The model under review builds one solid part; all positions refer to its coordinate system, in mm. A direction names the side the tool comes from. Round coordinates to 2 decimals unless told otherwise and drop trailing zeros. Order: outer loops, then holes, each group sorted by start corner. A loop starts at its lowest first (then second) coordinate and runs counter-clockwise, first axis right, second up. Notation, with made-up numbers: (-7, 78.5) -> (23, 78.5) arc R26 ccw to (23, 116.5) -> close; hole circle Ø4 at (-13, -16). An arc over 180 degrees is marked (long way). Use a Markdown table: item, result. Add a question column.
Autodesk Inventor part; units mm, degrees
ref_plane "YZ Plane" through (0, 0, 0) normal (1, 0, 0) x (0, 1, 0)
ref_plane "XZ Plane" through (0, 0, 0) normal (0, 1, 0) x (-1, 0, 0)
ref_plane "XY Plane" through (0, 0, 0) normal (0, 0, 1) x (1, 0, 0)
sketch "Sketch1" plane through (0, 0, 0) normal (0, 1, 0) x (-1, 0, 0)
  circle A0 centre (0, 0) radius 1
  circle A1 centre (0, 0) radius 2
  line L0 (2, 0) -> (-2, 0)
  line L1 (-2, 0) -> (-2, -8.25)
  line L2 (-2, -8.25) -> (2, -8.25)
  line L3 (2, -8.25) -> (2, 0)
  line L4 (2, -8.25) -> (4, -8.25)
  line L5 (4, -8.25) -> (4, -6.25)
  line L6 (4, -6.25) -> (2, -6.25)
  line L7 (2, -6.25) -> (2, -8.25)
  line L8 (-2, -8.25) -> (-4, -8.25)
  line L9 (-4, -8.25) -> (-4, -6.25)
  line L10 (-4, -6.25) -> (-2, -6.25)
  line L11 (-2, -6.25) -> (-2, -8.25)
  line L12 (0, 0) -> (0, -14.5)
  line L13 (0, 0) -> (14.5, 0) construction
  circle A2 centre (0, -14.5) radius 1
  circle A3 centre (0, -14.5) radius 2
  line L14 (2, -8.25) -> (-2, -8.25)
  line L15 (-2, -8.25) -> (-2, -14.5)
  line L16 (-2, -14.5) -> (2, -14.5)
  line L17 (2, -14.5) -> (2, -8.25)
  point P0 (-2, -6.25)
  point P1 (2, -6.25)
  point P2 (2, -14.5)
  dimension "d1" = 4
  dimension "d25" = 4
  dimension "d0" = 2
  dimension "d2" = 8.25
  dimension "d3" = 2
  dimension "d4" = 2
  dimension "d5" = 2
  dimension "d6" = 2
  dimension "d22" = 14.5
  dimension "d23" = 90
  dimension "d24" = 2
extrude "Extrusion1" add sketch "Sketch1" along normal blind 2 contours L0 A1 L12 A0 | A0 L0 A1 | A0 L12 A1 L0 | L3 L2 L12 A1 | A1 L12 L2 L1 | L6 L5 L4 L3 | L1 L8 L9 L10 | L12 A3 L15 L2 | L2 L17 A3 L12 | A3 L16 A2 L12 | L12 A2 L16 A3 | A3 L16 A2
sketch "Sketch2" plane through (0, 2, 0) normal (0, 1, 0) x (1, 0, 0)
  line L0 (-4, 6.25) -> (-2, 6.25)
  line L1 (4, 8.25) -> (-4, 8.25)
  line L2 (-4, 6.25) -> (-2, 6.25)
  line L3 (-2, 6.25) -> (-2, 8.25)
  line L4 (-2, 8.25) -> (-4, 8.25)
  line L5 (-4, 8.25) -> (-4, 6.25)
  line L6 (4, 6.25) -> (2, 6.25)
  line L7 (2, 6.25) -> (2, 8.25)
  line L8 (2, 8.25) -> (4, 8.25)
  line L9 (4, 8.25) -> (4, 6.25)
  point P0 (0, 0)
  point P1 (-4, 8.25)
  point P2 (-2, 6.25)
  dimension "d9" = 2
  dimension "d10" = 2
extrude "Extrusion2" add sketch "Sketch2" along normal blind 4.5
sketch "Sketch3" plane through (4, 0, -8.25) normal (0, 0, -1) x (-1, 0, 0)
  line L0 (2, 6.5) -> (0, 6.5)
  line L1 (2, 6.5) -> (2, 6)
  line L2 (2, 2) -> (2, 6.5)
  line L3 (2, 6) -> (6, 6)
  line L4 (2, 6) -> (3, 6)
  line L5 (3, 6) -> (3, 7)
  line L6 (3, 7) -> (2, 7)
  line L7 (2, 7) -> (2, 6)
  line L8 (6, 6) -> (5, 6)
  line L9 (5, 6) -> (5, 7)
  line L10 (5, 7) -> (6, 7)
  line L11 (6, 7) -> (6, 6)
  line L12 (2, 7) -> (0, 6.5)
  line L13 (8, 0) -> (8, 6.5)
  line L14 (6, 7) -> (8, 6.5)
  line L15 (8, 6.5) -> (6, 6.5)
  line L16 (0, 6.5) -> (2, 6.5)
  point P0 (4, 0)
  dimension "d13" = 0.5
  dimension "d14" = 4
  dimension "d15" = 1
  dimension "d16" = 1
  dimension "d17" = 1
  dimension "d18" = 1
extrude "Extrusion3" add sketch "Sketch3" against normal blind 2
fillet "Fillet1" radius 1.5 2 edges at (4, 6.5, -7.25) (-4, 6.5, -7.25)
fillet "Fillet2" radius 1.5 4 edges at (-2, 1, -6.25) (2, 1, -6.25) (-2, 1, -8.25) (2, 1, -8.25)
properties part number "leg_wire_holder"
Q1. Draft analysis for pull direction Z (two halves, no side actions). For faces 6 (the face through (2.45, 1.01, -5.82)), 7 (the face through (-1.5, 6, -7.3)), 8 (the face through (0.217, 0.986, -13.524)), state which applies: released by +Z, released by -Z, zero draft, split by the parting line, or undercut.
Q2. Add section C-C, the plane z = -6.5. Give the boundary of the cut face in (x, y), then the cut area to 3 significant figures.
Q3. Add section B-B, the plane x = 0. Give the boundary of the cut face in (y, z), then the cut area to 3 significant figures.
Q4. To check wall thickness, follow line 1 along Z through (x, y) = (0, 0.8); line 2 along X through (y, z) = (0.8, 0); line 3 along X through (y, z) = (4, -8). State the ranges of each line that lie inside material, in increasing order.
Q5. Add section A-A, the plane y = 2.25. Give the boundary of the cut face in (x, z).
Q6. For pin 1 (3 mm diameter, centred on y = 2.5, z = -12.5, fed in from -X); pin 2 (3 mm diameter, centred on x = 1.5, z = -2.5, fed in from +Y); pin 3 (0.5 mm diameter, centred on y = 6.5, z = -7.5, fed in from -X); pin 4 (1.8 mm diameter, centred on x = 0, z = 0, fed in from -Y), all flat-tipped, find the tip position at first contact; note any pin that passes through.
Q7. Add section D-D, the plane x = 1.75. Give the boundary of the cut face in (y, z).
Q8. For faces 1 (the face through (1.5, 6, -7.3)), 2 (the face through (2, 1, -2)), 3 (the face through (-2, 1, -12)), 4 (the face through (-1, 6.5, -7.3)), 5 (the face through (-2, 1, -2)), list the 3-axis set-ups (+Z, -Z, +X, -X, +Y, -Y) from which the entire face can be reached by the end or side of a thin tool; tool diameter is ignored.
Return value:
| question | item | result |
|---|---|---|
| 1 | face 6 | released by +Z |
| 1 | face 7 | zero draft |
| 1 | face 8 | undercut |
| 2 | outline | (-4, 0) -> (4, 0) -> (4, 5.33) arc R1.5 ccw to (2.86, 6.78) -> (2, 7) -> (1, 7) -> (1, 6) -> (2, 6) -> (2, 2) -> (-2, 2) -> (-2, 6) -> (-1, 6) -> (-1, 7) -> (-2, 7) -> (-2.86, 6.78) arc R1.5 ccw to (-4, 5.33) -> close |
| 2 | area | 36.5 mm² |
| 3 | outline | (0, -16.5) -> (2, -16.5) -> (2, -15.5) -> (0, -15.5) -> close; (0, -13.5) -> (2, -13.5) -> (2, -1) -> (0, -1) -> close; (0, 1) -> (2, 1) -> (2, 2) -> (0, 2) -> close |
| 3 | area | 29.0 mm² |
| 4 | line 1 | -16.5 to -15.5, -13.5 to -1, 1 to 2 |
| 4 | line 2 | -2 to -1, 1 to 2 |
| 4 | line 3 | -4 to -2, 2 to 4 |
| 5 | outline | (-4, -8.25) -> (-2, -8.25) -> (-2, -6.25) -> (-4, -6.25) -> close; (2, -8.25) -> (4, -8.25) -> (4, -6.25) -> (2, -6.25) -> close |
| 6 | pin 1 | x = -2 |
| 6 | pin 2 | y = 2 |
| 6 | pin 3 | x = -3.68 |
| 6 | pin 4 | through |
| 7 | outline | (0, -15.47) -> (2, -15.47) -> (2, 0.97) -> (0, 0.97) -> close; (6, -8.25) -> (7, -8.25) -> (7, -6.25) -> (6, -6.25) -> close |
| 8 | face 1 | +Z, -Z |
| 8 | face 2 | +Z, +X, +Y, -Y |
| 8 | face 3 | -Z, -X, +Y, -Y |
| 8 | face 4 | +Z, -Z, +Y |
| 8 | face 5 | +Z, -X, +Y, -Y |
